from build123d import *

# Parameters (mm, degrees)
F0_W     = 48
F0_H     = 48
F1_DEPTH = 48
F2_R     = 8
F3_DEPTH = 7
F3_TAPER = -3
F4_R     = 19
F5_DEPTH = 12


with BuildPart() as f1:
    # F0 (on Front) → F1 (new body)
    with BuildSketch(Plane.XZ):
        Rectangle(F0_W, F0_H)
    extrude(amount=F1_DEPTH)

    # F2 (on Front) → F3 (join)
    with BuildSketch(Plane.XZ):
        with Locations((-11.5896230564, 11.2924538553)):
            Circle(F2_R)
        with Locations((11.8867922574, 11.2924538553)):
            Circle(F2_R)
        with Locations((11.8867922574, -11.5896230564)):
            Circle(F2_R)
        with Locations((-11.5896230564, -11.5896230564)):
            Circle(F2_R)
    extrude(amount=F3_DEPTH, taper=F3_TAPER)

    # F4 (on Front) → F5 (join)
    with BuildSketch(Plane.XZ):
        Circle(F4_R)
    extrude(amount=-F5_DEPTH)


solid = f1.part
Build history of the part. All positions in model axes, mm. A direction names the side the tool comes from. Round coordinates to 2 decimals unless told otherwise and drop trailing zeros. Write each loop counter-clockwise with the first axis right and the second up, starting at its lowest first coordinate (ties: lowest second). Pieces come first, ordered by that corner, then holes. Notation, with made-up numbers: M 17,-9.75 L 62,-9.75 A22 ccw 62,19.25 Z; hole C -15.75,-30.5 d3. An arc over 180 degrees is marked long. Answer as a JSON object with one key per item and string values. Group by question number.
(1) Cut at A-A (z = 0). Give the cut face in (x, y), and give its area (3 significant figures).
(2) Which spindle directions (+Z, -Z, +X, -X, +Y, -Y) get a long thin tool onto all of the face, cutting with end or side? Do faces 1 (the flat face through (-24, -24, 0)), 2 (the cylindrical face through (8.767, 5.916, -16.856)). Say none if no direction does.
(3) Cut at B-B (x = 0). Give the cut face in (y, z).
(4) Drill centre lines: L1, parallel to Y at x = 16, z = -15; L2, parallel to Z at x = -0.5, y = 2. Where is each one in solid material? Low to high.
Responses:
{
 "1": {"outline": "M -24,-48 L 24,-48 L 24,0 L 19,0 L 19,12 L -19,12 L -19,0 L -24,0 Z", "area": "2,760 mm2"},
 "2": {"face 1": "+Z, -Z, -X, +Y, -Y", "face 2": "+Y"},
 "3": {"outline": "M -48,-24 L 0,-24 L 0,-19 L 12,-19 L 12,19 L 0,19 L 0,24 L -48,24 Z"},
 "4": {"L1": "y = -48 to 0", "L2": "z = -18.99 to 18.99"}
}
